Work out the finished part from the listing and answer in its coordinate system (mm). Give positions to 0.01 mm unless a question says otherwise; leave off trailing zeros. Loops run counter-clockwise (first coordinate to the right, second up) from the corner with the lowest first, then second, coordinate; pieces in that order, holes last. Notation, with made-up numbers: M 58,-5.5 L 102,-5.5 A9 cw 102,3.5 Z; hole C -23.75,80 d3. An arc over 180 degrees is marked long. Answer as a JSON object with one key per item and string values. Group by question number.
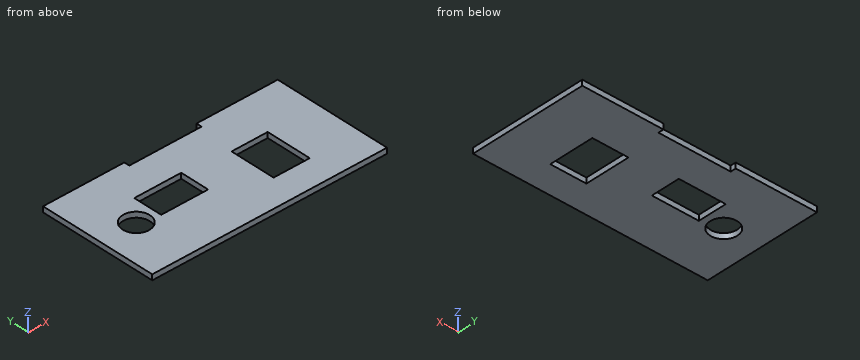
```python
from build123d import *

# Parameters (mm, degrees)
ESBO_O2_R                = 7.5
ESBO_O2_W                = 20
ESBO_O2_H                = 25
ESBO_O2_W_2              = 26
ESBO_O2_H_2              = 16
RESSALTO_EXTRUS_O1_DEPTH = 3


with BuildPart() as part:
    # Esboço2 → Ressalto-extrusão1 (new body)
    with BuildSketch(Plane.XY):
        Polygon((-50.047132184, 49.044084736), (-95.047132184, 49.044084736), (-95.047132184, -15.955915264), (34.952867816, -15.955915264), (34.952867816, 49.044084736), (-10.047132184, 49.044084736), (-10.047132184, 46.044084736), (-50.047132184, 46.044084736), align=None)
        with Locations((-75.047132184, 15.044084736)):
            Circle(ESBO_O2_R, mode=Mode.SUBTRACT)
        with Locations((-2.954931, 12.544084736)):
            Rectangle(ESBO_O2_W, ESBO_O2_H, mode=Mode.SUBTRACT)
        with Locations((-51.047132184, 20.044084736)):
            Rectangle(ESBO_O2_W_2, ESBO_O2_H_2, mode=Mode.SUBTRACT)
    extrude(amount=-RESSALTO_EXTRUS_O1_DEPTH)


solid = part.part
```
Item 1: Find the intervals of material crossed by probe 1 along X at (y, z) = (7, -1.5); probe 2 along Y at (x, z) = (-41.5, -2.1); probe 3 along X at (y, z) = (25.5, -2.1), in increasing order. Write a range as [from, to].
Item 2: A cutting plane is placed at A-A (x = -6.5). Determine the outline of the cut face in (y, z), and give its area (3 significant figures).
Item 3: A cutting plane is placed at C-C (x = -62). Determine the outline of the cut face in (y, z), and give its area (3 significant figures).
Item 4: A cutting plane is placed at D-D (x = -33.5). Determine the outline of the cut face in (y, z).
Item 5: A cutting plane is placed at B-B (z = -0.7). Determine the outline of the cut face in (x, y).
The answers:
{
 "1": {"probe 1": "x = [-95.05, -12.95], [7.05, 34.95]", "probe 2": "y = [-15.96, 12.04], [28.04, 46.04]", "probe 3": "x = [-95.05, -64.05], [-38.05, 34.95]"},
 "2": {"outline": "M -15.96,-3 L 0.04,-3 L 0.04,0 L -15.96,0 Z; M 25.04,-3 L 49.04,-3 L 49.04,0 L 25.04,0 Z", "area": "120 mm^2"},
 "3": {"outline": "M -15.96,-3 L 12.04,-3 L 12.04,0 L -15.96,0 Z; M 28.04,-3 L 49.04,-3 L 49.04,0 L 28.04,0 Z", "area": "147 mm^2"},
 "4": {"outline": "M -15.96,-3 L 46.04,-3 L 46.04,0 L -15.96,0 Z"},
 "5": {"outline": "M -95.05,-15.96 L 34.95,-15.96 L 34.95,49.04 L -10.05,49.04 L -10.05,46.04 L -50.05,46.04 L -50.05,49.04 L -95.05,49.04 Z; hole C -75.05,15.04 d15; hole M -64.05,12.04 L -38.05,12.04 L -38.05,28.04 L -64.05,28.04 Z; hole M -12.95,0.04 L 7.05,0.04 L 7.05,25.04 L -12.95,25.04 Z"}
}
